Design review of the part built by this model. Coordinates are the model's own, in mm. A direction names the side the tool comes from. Round coordinates to 2 decimals unless told otherwise and drop trailing zeros. Order: outer loops, then holes, each group sorted by start corner. A loop starts at its lowest first (then second) coordinate and runs counter-clockwise, first axis right, second up.
from build123d import *

# Parameters (mm, degrees)
SKETCH1_W           = 588
SKETCH1_H           = 22.5
BOSS_EXTRUDE1_DEPTH = 2.5
SKETCH2_W           = 588
SKETCH2_H           = 2.5
BOSS_EXTRUDE2_DEPTH = 20
FILLET1_R           = 1


with BuildPart() as part:
    # Sketch1 → Boss-Extrude1 (new body)
    with BuildSketch(Plane(origin=(0, 0, 0), x_dir=(1, 0, 0), z_dir=(0, 1, 0))):
        Rectangle(SKETCH1_W, SKETCH1_H)
    extrude(amount=BOSS_EXTRUDE1_DEPTH)

    # Sketch2 → Boss-Extrude2 (add)
    with BuildSketch(Plane(origin=(0, 2.5, 0), x_dir=(1, 0, 0), z_dir=(0, 1, 0))):
        with Locations((0, 10)):
            Rectangle(SKETCH2_W, SKETCH2_H)
    extrude(amount=BOSS_EXTRUDE2_DEPTH)

    # Fillet1
    fillet1_edges = [part.edges().sort_by_distance(p)[0] for p in [
        (0, 2.5, 11.25),
        (0, 2.5, -8.75),
        (0, 22.5, -8.75),
        (0, 22.5, -11.25),
        (0, 0, 11.25),
        (0, 0, -11.25),
    ]]
    fillet(fillet1_edges, radius=FILLET1_R)


solid = part.part
1) Take a section at B-B on z = -3. Give the boundary of the cut face in (x, y).
Results:
outline: (-294, 0) - (294, 0) - (294, 2.5) - (-294, 2.5) - close
2) To check wall thickness, follow line 1 along Y through (x, z) = (53, -4.75); line 2 along Z through (x, y) = (262, 5.25); line 3 along Y through (x, z) = (-86, -9.5). State the ranges of each line that lie inside material, in increasing order.
Results:
line 1: y = 0 to 2.5
line 2: z = -11.25 to -8.75
line 3: y = 0 to 22.47
3) Take a section at C-C on y = 8.5. Give the boundary of the cut face in (x, z).
Results:
outline: (-294, -11.25) - (294, -11.25) - (294, -8.75) - (-294, -8.75) - close
4) Clearance check with flat-ended pins moving along their axes: P1, Ø1.5, axis at x = -66, z = 3.5, coming from the +Y side; P2, Ø3, axis at x = -61.5, y = 19.5, coming from the +Z side. State where each tip first meets the part, or that it passes through.
Results:
P1: stops at y = 2.5
P2: stops at z = -8.75
5) For faces 1 (the face through (-4, 12, -8.75)), 2 (the face through (-4, 11, -11.25)), list the 3-axis set-ups (+Z, -Z, +X, -X, +Y, -Y) from which the entire face can be reached by the end or side of a thin tool; tool diameter is ignored.
Results:
face 1: +Z, +X, -X, +Y
face 2: -Z, +X, -X, +Y, -Y
6) Take a section at A-A on x = -247. Give the boundary of the cut face in (y, z).
Results:
outline: (0, -10.25) arc R1 ccw to (1, -11.25) - (21.5, -11.25) arc R1 ccw to (22.5, -10.25) - (22.5, -9.75) arc R1 ccw to (21.5, -8.75) - (3.5, -8.75) arc R1 cw to (2.5, -7.75) - (2.5, 10.25) arc R1 ccw to (1.5, 11.25) - (1, 11.25) arc R1 ccw to (0, 10.25) - close
